Build history of the part. All positions in model axes, mm. A direction names the side the tool comes from. Give positions to 0.01 mm unless a question says otherwise; leave off trailing zeros. Order: outer loops, then holes, each group sorted by start corner. A loop starts at its lowest first (then second) coordinate and runs counter-clockwise, first axis right, second up. Notation, with made-up numbers: (29.25, 9) -> (34.25, 9) arc R32 ccw to (34.25, 45) -> close; hole circle Ø7 at (18, 61). An arc over 180 degrees is marked (long way). One line per item, written item: value. Start each with the question number.
(1) Saw through at B-B on y = 29. Give the cut face in (x, z), plus the area to 3 significant figures.
(2) Saw through at A-A on x = 0. Give the cut face in (y, z) (3 decimals), plus the area to 3 significant figures.
(3) Pin check, flat tips, straight feed: pin 1 (6.5 mm diameter, centred on x = -0.5, z = 98.5, fed in from -Y); pin 2 (9.5 mm diameter, centred on x = 2, y = 32.5, fed in from -Z). Stop position of each tip, or through.
(4) Which spindle directions (+Z, -Z, +X, -X, +Y, -Y) get a long thin tool onto all of the face, cutting with end or side? Do faces 5 (the flat face through (3, 3, 113)), 6 (the flat face through (0, 29, 52)), 7 (the flat face through (0, 50, 110)). Say none if no direction does.
(5) Probe line 1 (Y direction, x = 18.5, z = 170) (3 decimals); line 2 (Y direction, x = 0, z = 39); line 3 (Z direction, x = 6.5, y = 9). List the from-to ranges inside material, lowest first.
(6) Two-plate mould, pull along X, no slides. Class faces 1 (the flat face through (0, 6, 113)), 2 (the cylindrical face through (2.07, 19.677, 25.636)), 3 (the flat face through (-8, 20, 0)), 4 (the flat face through (-32.5, 25, 110)): +X half, -X half, draft (parallel to the pull), parting line (faces both ways), or undercut.
```python
from build123d import *

# Parameters (mm, degrees)
SKETCH1_W                = 65
SKETCH1_H                = 50
BALSA_BLOCK_DEPTH        = 223
SKETCH2_W                = 6
SKETCH2_H                = 6
SCREW_EYE_SLOT_DEPTH     = 231.835980731
SKETCH3_R                = 9.55
CO2_CARTRIDGE_HOLE_DEPTH = 52
SKETCH4_R                = 1.525
AXLE_HOLE_CUT_OUT_DEPTH  = 238.60050505


with BuildPart() as part:
    # Sketch1 → Balsa Block (new body)
    with BuildSketch(Plane.XY):
        with Locations((0, 25)):
            Rectangle(SKETCH1_W, SKETCH1_H)
    extrude(amount=BALSA_BLOCK_DEPTH)

    # Sketch2 → Screw Eye Slot (cut, through all)
    with BuildSketch(Plane.XY.offset(223)):
        with Locations((0, 3)):
            Rectangle(SKETCH2_W, SKETCH2_H)
    extrude(amount=-SCREW_EYE_SLOT_DEPTH, mode=Mode.SUBTRACT)

    # Sketch3 → CO2 Cartridge Hole (cut)
    with BuildSketch(Plane(origin=(0, 0, 0), x_dir=(-1, 0, 0), z_dir=(0, 0, -1))):
        with Locations((0, 29)):
            Circle(SKETCH3_R)
    extrude(amount=-CO2_CARTRIDGE_HOLE_DEPTH, mode=Mode.SUBTRACT)

    # Sketch4 → Axle Hole Cut Out (cut, through all)
    with BuildSketch(Plane(origin=(32.5, 0, 0), x_dir=(0, 0, -1), z_dir=(1, 0, 0))):
        with Locations((-170, 10)):
            Circle(SKETCH4_R)
        with Locations((-35, 10)):
            Circle(SKETCH4_R)
    extrude(amount=-AXLE_HOLE_CUT_OUT_DEPTH, mode=Mode.SUBTRACT)


solid = part.part
```
Results below:
1. outline: (-32.5, 0) -> (-9.55, 0) -> (-9.55, 52) -> (9.55, 52) -> (9.55, 0) -> (32.5, 0) -> (32.5, 223) -> (-32.5, 223) -> close
1. area: 13,500 mm²
2. outline: (6, 0) -> (19.45, 0) -> (19.45, 52) -> (38.55, 52) -> (38.55, 0) -> (50, 0) -> (50, 223) -> (6, 223) -> close; hole circle Ø3.05 at (10, 35); hole circle Ø3.05 at (10, 170)
2. area: 8,800 mm²
3. pin 1: stops at y = 0
3. pin 2: stops at z = 52
4. face 5: +Z, -Z, -Y
4. face 6: -Z
4. face 7: +Z, -Z, +X, -X, +Y
5. line 1: y = 0 to 8.475, 11.525 to 50
5. line 2: y = 6 to 19.45, 38.55 to 50
5. line 3: z = 0 to 33.85, 36.15 to 168.85, 171.15 to 223
6. face 1: undercut
6. face 2: undercut
6. face 3: draft
6. face 4: -X half
